Work out the finished part from the listing and answer in its coordinate system (mm). Round coordinates to 2 decimals unless told otherwise and drop trailing zeros. Loops run counter-clockwise (first coordinate to the right, second up) from the corner with the lowest first, then second, coordinate; pieces in that order, holes last.
Autodesk Inventor part; units mm, degrees
ref_plane "YZ Plane" through (0, 0, 0) normal (1, 0, 0) x (0, 1, 0)
ref_plane "XZ Plane" through (0, 0, 0) normal (0, 1, 0) x (-1, 0, 0)
ref_plane "XY Plane" through (0, 0, 0) normal (0, 0, 1) x (1, 0, 0)
sketch "Sketch1" plane through (0, 0, 0) normal (0, 1, 0) x (-1, 0, 0)
  line L0 (12.7, 12.7) -> (-12.7, 12.7)
  line L1 (-12.7, 12.7) -> (-12.7, -12.7)
  line L2 (-12.7, -12.7) -> (12.7, -12.7)
  line L3 (12.7, -12.7) -> (12.7, 12.7)
  line L4 (12.7, 12.7) -> (-12.7, -12.7) construction
  line L5 (-12.7, 12.7) -> (12.7, -12.7) construction
  line L6 (9.525, 9.525) -> (-9.525, 9.525)
  line L7 (-9.525, 9.525) -> (-9.525, -9.525)
  line L8 (-9.525, -9.525) -> (9.525, -9.525)
  line L9 (9.525, -9.525) -> (9.525, 9.525)
  line L10 (9.525, 9.525) -> (-9.525, -9.525) construction
  line L11 (-9.525, 9.525) -> (9.525, -9.525) construction
  point P0 (0, 0)
  dimension "d0" = 25.4
  dimension "d1" = 3.175
extrude "Extrusion1" add sketch "Sketch1" along normal blind 1168.4
properties part number "1x46-rectangular"
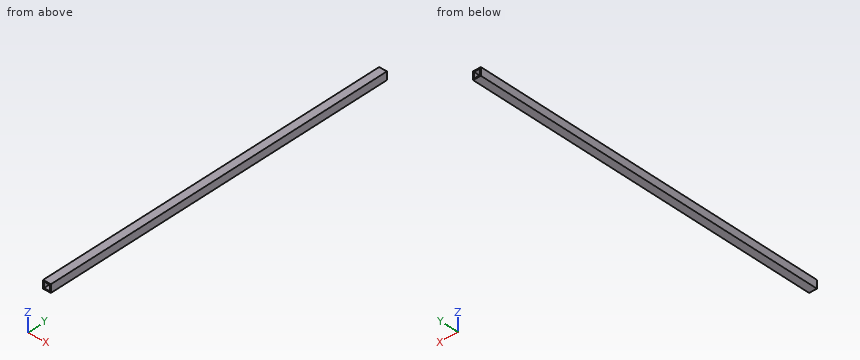
Item 1: Section A-A, the plane x = -5 is taken. Give the vertices of the cut face in (y, z) (3 decimals).
Item 2: This flat-tipped pin is pushed along its axis until it touches: P1, Ø10, axis at x = 4, z = 2, coming from the -Y side. Where does it stop, or does it pass through?
Item 3: A straight line is drawn through the part: line 1 (X direction, y = 203, z = -4.25) (3 decimals). Find the intervals that lie inside material, in ascending order.
Item 4: Section B-B, the plane z = -1.5 is taken. Give the vertices of the cut face in (x, y) (3 decimals), plus the area to 3 significant figures.
Item 5: Section C-C, the plane y = 982 is taken. Give the vertices of the cut face in (x, z) (3 decimals), plus the area to 3 significant figures.
Answer below:
1. outline: (0, -12.7) - (1168.4, -12.7) - (1168.4, -9.525) - (0, -9.525) - close; (0, 9.525) - (1168.4, 9.525) - (1168.4, 12.7) - (0, 12.7) - close
2. P1: passes through
3. line 1: x = -12.7 to -9.525, 9.525 to 12.7
4. outline: (-12.7, 0) - (-9.525, 0) - (-9.525, 1168.4) - (-12.7, 1168.4) - close; (9.525, 0) - (12.7, 0) - (12.7, 1168.4) - (9.525, 1168.4) - close
4. area: 7,420 mm2
5. outline: (-12.7, -12.7) - (12.7, -12.7) - (12.7, 12.7) - (-12.7, 12.7) - close; hole (-9.525, -9.525) - (9.525, -9.525) - (9.525, 9.525) - (-9.525, 9.525) - close
5. area: 282 mm2
